Part print with two shaded views. Sizes in mm from the minimum x, y, z corner. A direction names the side the tool comes from. Round coordinates to 2 decimals unless told otherwise and drop trailing zeros. Write each loop counter-clockwise with the first axis right and the second up, starting at its lowest first coordinate (ties: lowest second). Pieces come first, ordered by that corner, then holes. Notation, with made-up numbers: (-1.75, 16.25) -> (10.25, 16.25) arc R18 cw to (10.25, 38.25) -> close; hole circle Ø8 at (85, 10). An arc over 180 degrees is marked (long way). Return JSON: item names as keys, results as strings.
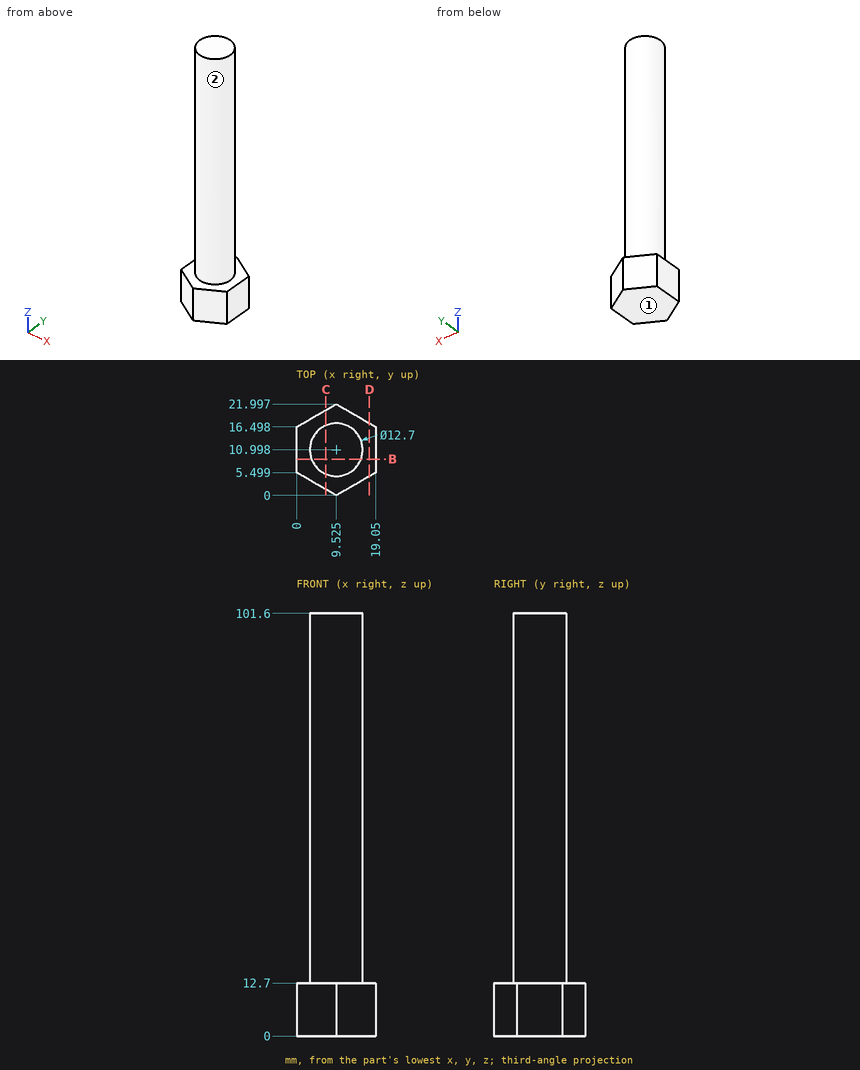
Q1. Pin check, flat tips, straight feed: pin 1 Ø12 at (y, z) = (6, 43) entering from -X (1 decimal); pin 2 Ø1.5 at (x, y) = (17, 3.5) entering from +Z; pin 3 Ø5 at (x, y) = (7.5, 4) entering from -Z; pin 4 Ø12 at (y, z) = (6, 50.5) entering from +X (1 decimal). Stop position of each tip, or through.
Verdict:
{"pin 1": "stops at x = 3.2", "pin 2": "stops at z = 12.7", "pin 3": "stops at z = 0", "pin 4": "stops at x = 15.9"}
Q2. Saw through at D-D on x = 17.5. List the corners of the cut face in (y, z) (1 decimal), then the cut area to 3 significant figures.
Verdict:
{"outline": "(4.6, 0) -> (17.4, 0) -> (17.4, 12.7) -> (4.6, 12.7) -> close", "area": "162 mm²"}
Q3. Saw through at B-B on y = 8.75. List the corners of the cut face in (x, z), then the cut area to 3 significant figures.
Verdict:
{"outline": "(0, 0) -> (19.05, 0) -> (19.05, 12.7) -> (15.46, 12.7) -> (15.46, 101.6) -> (3.59, 101.6) -> (3.59, 12.7) -> (0, 12.7) -> close", "area": "1,300 mm²"}
Q4. Saw through at C-C on x = 7. List the corners of the cut face in (y, z) (1 decimal).
Verdict:
{"outline": "(1.5, 0) -> (20.5, 0) -> (20.5, 12.7) -> (16.8, 12.7) -> (16.8, 101.6) -> (5.2, 101.6) -> (5.2, 12.7) -> (1.5, 12.7) -> close"}
Q5. Wall check: L1, parallel to Z at x = 7.25, y = 17.25; L2, parallel to Y at x = 10, z = 44.5; L3, parallel to X at y = 11.5, z = 91 (1 decimal). Give the ranges that are in metal, low to high.
Verdict:
{"L1": "z = 0 to 12.7", "L2": "y = 4.67 to 17.33", "L3": "x = 3.2 to 15.9"}
Q6. 3-axis set-ups, long thin cutter, end or side, ignore diameter. For the marked faces 1 and 2: which of +Z, -Z, +X, -X, +Y, -Y reach the whole face in a straight line?
Verdict:
{"face 1": "-Z, +X, -X, +Y, -Y", "face 2": "+Z"}
